Geometry: final body of the model. Coordinates: model frame, mm. Face numbers are marked on the shaded views. A direction names the side the tool comes from. Coordinates: 2 decimals unless noted, no trailing zeros. Write each loop counter-clockwise with the first axis right and the second up, starting at its lowest first coordinate (ties: lowest second). Pieces come first, ordered by that corner, then holes. Notation, with made-up numbers: (42, 52) -> (46, 52) arc R30 ccw to (46, 77) -> close; hole circle Ø6 at (89, 47). An arc over 180 degrees is marked (long way). Answer as a JSON object with one key per item and string values. Group by question number.
```python
from build123d import *

# Parameters (mm, degrees)
SKETCH_1_R               = 11.5
EXTRUDE_1_DEPTH          = 0.5
SKETCH_2_R               = 9.295
EXTRUDE_2_DEPTH          = 11
SKETCH_8_R               = 7.5
EXTRUDE_4_DEPTH          = 10
CUT_EXTRUDE_3_DEPTH      = 11
SKETCH_3_R               = 11.5
EXTRUDE_3_DEPTH          = 1
SKETCH_6_R               = 3
CUT_EXTRUDE_2_DEPTH      = 10.5
CUT_EXTRUDE_2_DEPTH_BACK = 14
PATTERN_CIRCULAR_2_COUNT = 30


with BuildPart() as part:
    # 草圖1 → 填料-伸長1 (new body, symmetric)
    with BuildSketch(Plane.XY):
        Circle(SKETCH_1_R)
    extrude(amount=EXTRUDE_1_DEPTH, both=True)

    # 草圖2 → 填料-伸長2 (add)
    with BuildSketch(Plane.XY.offset(0.5)):
        Circle(SKETCH_2_R)
    extrude(amount=EXTRUDE_2_DEPTH)

    # 草圖8 → 填料-伸長4 (add)
    with BuildSketch(Plane(origin=(0, 0, 0), x_dir=(-1, 0, 0), z_dir=(0, 0, -1))):
        Circle(SKETCH_8_R)
    extrude(amount=EXTRUDE_4_DEPTH)

    # 草圖7 → 除料-伸長3 (cut)
    with BuildSketch(Plane.XY.offset(11.5)):
        with BuildLine():
            ThreePointArc((-0.599687408, 9.27563475), (0, 8.695), (0.599687408, 9.27563475))
            ThreePointArc((0.599687408, 9.27563475), (0, 9.295), (-0.599687408, 9.27563475))
        make_face()
    cut_extrude_3 = extrude(amount=-CUT_EXTRUDE_3_DEPTH, mode=Mode.SUBTRACT)

    # 草圖3 → 填料-伸長3 (add)
    with BuildSketch(Plane.XY.offset(11.5)):
        Circle(SKETCH_3_R)
    extrude(amount=EXTRUDE_3_DEPTH)

    # 草圖6 → 除料-伸長2 (cut, two sides)
    with BuildSketch(Plane(origin=(0, 0, -0.5), x_dir=(-1, 0, 0), z_dir=(0, 0, -1))) as cut_extrude_2_sk:
        Circle(SKETCH_6_R)
    extrude(amount=CUT_EXTRUDE_2_DEPTH, mode=Mode.SUBTRACT)
    extrude(cut_extrude_2_sk.sketch, amount=-CUT_EXTRUDE_2_DEPTH_BACK, mode=Mode.SUBTRACT)

    # 環狀複製排列2: 除料-伸長3 ×30 about axis
    pattern_circular_2_axis = Axis((0, 0, 0), (0, 0, 1))
    for i in range(1, PATTERN_CIRCULAR_2_COUNT):
        add(cut_extrude_3.rotate(pattern_circular_2_axis, i * 360 / PATTERN_CIRCULAR_2_COUNT), mode=Mode.SUBTRACT)


solid = part.part
```
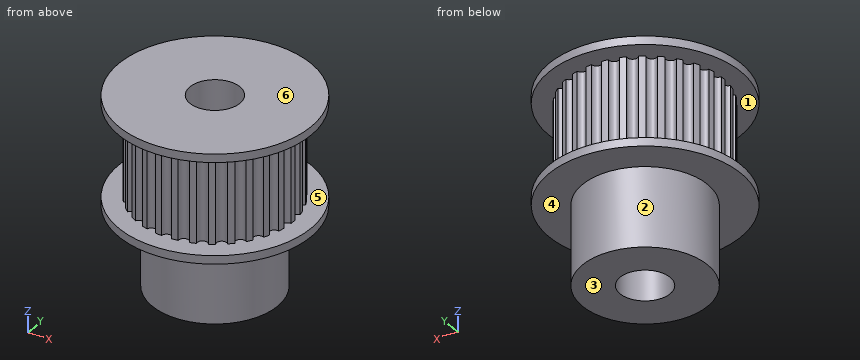
Item 1: Mould query, pull axis Z, two halves, no side actions, for the marked faces 4, 5 and 6. Classes: +Z half, -Z half, draft (parallel to the pull), parting line (faces both ways), or undercut.
Item 2: Set-up query: the marked faces 1, 2 and 3. Return all of +Z, -Z, +X, -X, +Y, -Y with unobstructed straight access to the full face (end or side cutting, diameter ignored); none if empty.
Item 3: Section B-B on x = 0. Output: boundary loops of the cut face in (y, z) (3 decimals).
Item 4: Section A-A on y = 0. Output: boundary loops of the cut face in (x, z) (3 decimals), then the cut area to 3 significant figures.
Item 5: Ray query, L1, parallel to X at y = 0, z = -2.25; L2, parallel to Y at x = 0, z = 3.5 (3 decimals); L3, parallel to X at y = 0, z = 6 (3 decimals). Return the intervals inside material, ascending. Write a range as [from, to].
Item 6: Contact query for flat-ended pins moving along their axis: pin 1 (4 mm diameter, centred on y = -5, z = 7, fed in from -X); pin 2 (1 mm diameter, centred on x = 2.5, z = 2, fed in from -Y); pin 3 (5 mm diameter, centred on x = 0, y = 0, fed in from +Z); pin 4 (5 mm diameter, centred on y = -7, z = -4.5, fed in from +X). Output: stop coordinate, or through.
Item 7: Section C-C on y = 9.75. Output: boundary loops of the cut face in (x, z), then the cut area to 3 significant figures.
Answer sheet:
{
 "1": {"face 4": "-Z half", "face 5": "undercut", "face 6": "+Z half"},
 "2": {"face 1": "none", "face 2": "-Z", "face 3": "-Z, +X, -X, +Y, -Y"},
 "3": {"outline": "(-11.5, -0.5) -> (-7.5, -0.5) -> (-7.5, -10) -> (-3, -10) -> (-3, 12.5) -> (-11.5, 12.5) -> (-11.5, 11.5) -> (-8.695, 11.5) -> (-8.695, 0.5) -> (-11.5, 0.5) -> close; (3, -10) -> (7.5, -10) -> (7.5, -0.5) -> (11.5, -0.5) -> (11.5, 0.5) -> (8.695, 0.5) -> (8.695, 11.5) -> (11.5, 11.5) -> (11.5, 12.5) -> (3, 12.5) -> close"},
 "4": {"outline": "(-11.5, -0.5) -> (-7.5, -0.5) -> (-7.5, -10) -> (-3, -10) -> (-3, 12.5) -> (-11.5, 12.5) -> (-11.5, 11.5) -> (-9.295, 11.5) -> (-9.295, 0.5) -> (-11.5, 0.5) -> close; (3, -10) -> (7.5, -10) -> (7.5, -0.5) -> (11.5, -0.5) -> (11.5, 0.5) -> (9.295, 0.5) -> (9.295, 11.5) -> (11.5, 11.5) -> (11.5, 12.5) -> (3, 12.5) -> close", "area": "258 mm^2"},
 "5": {"L1": "x = [-7.5, -3], [3, 7.5]", "L2": "y = [-8.695, -3], [3, 8.695]", "L3": "x = [-9.295, -3], [3, 9.295]"},
 "6": {"pin 1": "stops at x = -8.64", "pin 2": "stops at y = -8.95", "pin 3": "passes through", "pin 4": "stops at x = 6"},
 "7": {"outline": "(-6.1, -0.5) -> (6.1, -0.5) -> (6.1, 0.5) -> (-6.1, 0.5) -> close; (-6.1, 11.5) -> (6.1, 11.5) -> (6.1, 12.5) -> (-6.1, 12.5) -> close", "area": "24.4 mm^2"}
}
